Verification items for the finished model (mm, model axes). Coordinates: 2 decimals unless noted, no trailing zeros. Order: outer loops, then holes, each group sorted by start corner. A loop starts at its lowest first (then second) coordinate and runs counter-clockwise, first axis right, second up. Notation, with made-up numbers: (-4, -39.75) -> (13, -39.75) arc R16 cw to (13, -15.75) -> close; hole circle Ø5 at (24, -1). An arc over 180 degrees is marked (long way). Answer as CSV lines item,"result".
```python
from build123d import *

# Parameters (mm, degrees)
F0_W     = 279.4
F0_H     = 370.84
F1_DEPTH = 12.7
F3_DEPTH = 12.7
F4_START = -358.14
F4_DEPTH = 12.7


with BuildPart() as f1:
    # F0 (on Top) → F1 (new body)
    with BuildSketch(Plane.XY):
        Rectangle(F0_W, F0_H)
    extrude(amount=F1_DEPTH)

    # F2 (on face) → F3 (join)
    with BuildSketch(Plane(origin=(0, 185.42, 0), x_dir=(-1, 0, 0), z_dir=(0, 1, 0))):
        with BuildLine():
            Line((-139.7, -82.55), (-139.7, -95.25))
            Line((-139.7, -95.25), (139.7, -95.25))
            ThreePointArc((139.7, -95.25), (179.3299440444, -41.275), (139.7, 12.7))
            Line((139.7, 12.7), (139.7, 0))
            ThreePointArc((139.7, 0), (167.7143480452, -41.275), (139.7, -82.55))
            Line((139.7, -82.55), (-139.7, -82.55))
        make_face()
    extrude(amount=-F3_DEPTH)

    # F2 (on face) → F4 (join)
    with BuildSketch(Plane(origin=(0, 185.42, 0), x_dir=(-1, 0, 0), z_dir=(0, 1, 0)).offset(F4_START)):
        with BuildLine():
            Line((-139.7, -82.55), (-139.7, -95.25))
            Line((-139.7, -95.25), (139.7, -95.25))
            ThreePointArc((139.7, -95.25), (179.3299440444, -41.275), (139.7, 12.7))
            Line((139.7, 12.7), (139.7, 0))
            ThreePointArc((139.7, 0), (167.7143480452, -41.275), (139.7, -82.55))
            Line((139.7, -82.55), (-139.7, -82.55))
        make_face()
    extrude(amount=-F4_DEPTH)


solid = f1.part
```
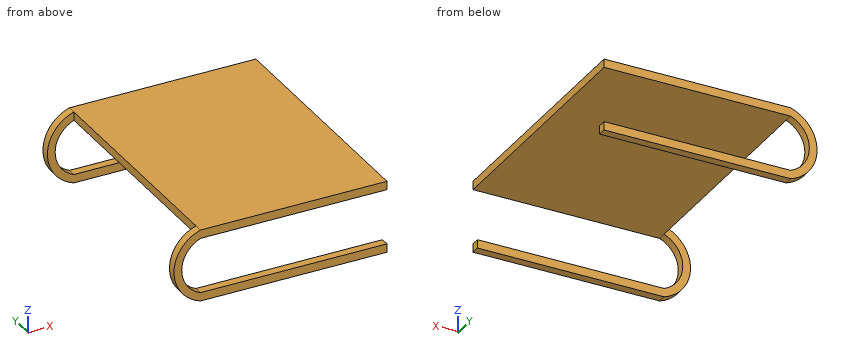
Item 1: Section check B-B, the plane z = -22.5. Record the boundary of the cut face in (x, y), plus the area to 3 significant figures.
Answer list:
outline,"(-176.12, -185.42) -> (-163.55, -185.42) -> (-163.55, -172.72) -> (-176.12, -172.72) -> close; (-176.12, 172.72) -> (-163.55, 172.72) -> (-163.55, 185.42) -> (-176.12, 185.42) -> close"
area,"319 mm2"
Item 2: Section check A-A, the plane x = 23. Record the boundary of the cut face in (y, z).
Answer list:
outline,"(-185.42, -95.25) -> (-172.72, -95.25) -> (-172.72, -82.55) -> (-185.42, -82.55) -> close; (-185.42, 0) -> (185.42, 0) -> (185.42, 12.7) -> (-185.42, 12.7) -> close; (172.72, -95.25) -> (185.42, -95.25) -> (185.42, -82.55) -> (172.72, -82.55) -> close"
Item 3: Section check C-C, the plane z = 5. Record the boundary of the cut face in (x, y).
Answer list:
outline,"(-155.3, -185.42) -> (139.7, -185.42) -> (139.7, 185.42) -> (-155.3, 185.42) -> (-155.3, 172.72) -> (-139.7, 172.72) -> (-139.7, -172.72) -> (-155.3, -172.72) -> close"
Item 4: Depth check by flat-ended pin: pin 1 Ø10 at (x, z) = (-55.5, -9.5) entering from +Y; pin 2 Ø14 at (y, z) = (-19, 6) entering from -X; pin 3 Ø3 at (x, y) = (34, -99) entering from -Z. Enter the tip coordinate at first touch or a pass-through.
Answer list:
pin 1,"through"
pin 2,"x = -139.7"
pin 3,"z = 0"
Item 5: Thickness scan on line 1 (Y direction, x = -29.5, z = -91); line 2 (Z direction, x = -109, y = -153.5); line 3 (X direction, y = -138, z = 0.5). Record the ranges inside material, lowest first.
Answer list:
line 1,"-185.42 to -172.72, 172.72 to 185.42"
line 2,"0 to 12.7"
line 3,"-139.7 to 139.7"
Item 6: Section check D-D, the plane z = -72.5. Record the boundary of the cut face in (x, y).
Answer list:
outline,"(-169.93, -185.42) -> (-154.88, -185.42) -> (-154.88, -172.72) -> (-169.93, -172.72) -> close; (-169.93, 172.72) -> (-154.88, 172.72) -> (-154.88, 185.42) -> (-169.93, 185.42) -> close"
